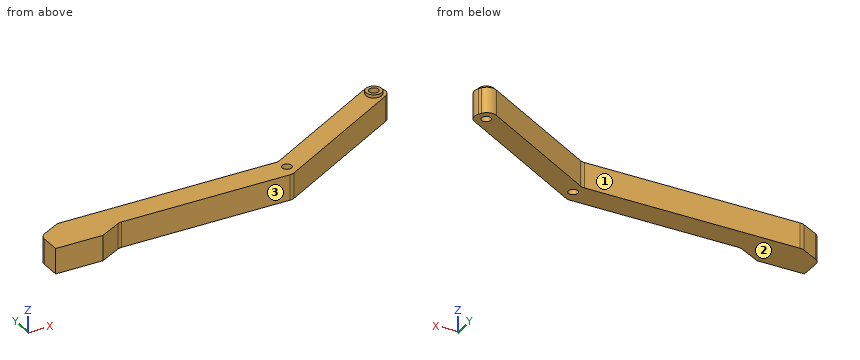
from build123d import *

# Parameters (mm, degrees)
SKETCH_1_R      = 1.5
EXTRUDE_1_DEPTH = 8
FILLET_1_R      = 3
SKETCH_2_R      = 2.5
SKETCH_2_R_2    = 1.5
EXTRUDE_2_DEPTH = 1


with BuildPart() as part:
    # 草图1 → 凸台-拉伸1 (new body)
    with BuildSketch(Plane.XY):
        Polygon((-7.5, 4), (-7.5, -4), (7.5, -4), (15, 0), (70, 0), (116.765371804, 27), (113.301270189, 33), (70, 8), (0, 8), align=None)
        with Locations((112.0368731, 28.27)):
            Circle(SKETCH_1_R, mode=Mode.SUBTRACT)
        with Locations((70.727461339, 4.42)):
            Circle(SKETCH_1_R, mode=Mode.SUBTRACT)
    extrude(amount=EXTRUDE_1_DEPTH)

    # 圆角1
    fillet_1_edges = [part.edges().sort_by_distance(p)[0] for p in [
        (-7.5, 4, 4),
        (0, 8, 4),
        (70, 8, 4),
        (113.301270189, 33, 4),
        (116.765371804, 27, 4),
        (70, 0, 4),
        (15, 0, 4),
    ]]
    fillet(fillet_1_edges, radius=FILLET_1_R)

    # 草图2 → 凸台-拉伸2 (add)
    with BuildSketch(Plane.XY.offset(8)):
        with Locations((112.0368731, 28.27)):
            Circle(SKETCH_2_R)
        with Locations((112.0368731, 28.27)):
            Circle(SKETCH_2_R_2, mode=Mode.SUBTRACT)
    extrude(amount=EXTRUDE_2_DEPTH)


solid = part.part
Check sheet for the modelled part. Datum: model origin and axes. Units: mm. Face numbers are marked on the shaded views. A direction names the side the tool comes from. Round coordinates to 2 decimals unless told otherwise and drop trailing zeros. Order: outer loops, then holes, each group sorted by start corner. A loop starts at its lowest first (then second) coordinate and runs counter-clockwise, first axis right, second up.
Q1. Scan lines: L1, parallel to Z at x = 38.5, y = 4; L2, parallel to Y at x = 1, z = 3.75; L3, parallel to X at y = 24, z = 5. Record each from-to range of solid material in increasing order.
Filled sheet:
L1: z = 0 to 8
L2: y = -4 to 8
L3: x = 97.71 to 111.57
Q2. Cross-section at A-A, the plane z = 5. Enter the section's corners in (x, y), plus the area to 3 significant figures.
Filled sheet:
outline: (-7.5, -4) - (7.5, -4) - (14.34, -0.35) arc R3 cw to (15.75, 0) - (69.2, 0) arc R3 ccw to (70.7, 0.4) - (114.17, 25.5) arc R3 ccw to (115.27, 29.6) - (114.8, 30.4) arc R3 ccw to (110.7, 31.5) - (70.7, 8.4) arc R3 cw to (69.2, 8) - (0.75, 8) arc R3 ccw to (-0.66, 7.65) - (-5.91, 4.85) arc R3 ccw to (-7.5, 2.2) - close; hole circle Ø3 at (70.73, 4.42); hole circle Ø3 at (112.04, 28.27)
area: 1,020 mm2
Q3. Cross-section at B-B, the plane y = 28.27. Enter the section's corners in (x, z), plus the area to 3 significant figures.
Filled sheet:
outline: (105.11, 0) - (110.54, 0) - (110.54, 9) - (109.54, 9) - (109.54, 8) - (105.11, 8) - close; (113.54, 0) - (115.66, 0) - (115.66, 8) - (114.54, 8) - (114.54, 9) - (113.54, 9) - close
area: 62.4 mm2
Q4. Set-up check for the marked faces 1, 2 and 3: record each of +Z, -Z, +X, -X, +Y, -Y from which the full face is reachable in a straight line by a thin tool's end or side.
Filled sheet:
face 1: +Z, -Z, -X, +Y
face 2: -Z, +X, -X, +Y, -Y
face 3: +Z, -Z, +X, -Y
Q5. Cross-section at D-D, the plane y = 21. Enter the section's corners in (x, z).
Filled sheet:
outline: (92.52, 0) - (106.37, 0) - (106.37, 8) - (92.52, 8) - close
Q6. Depth check by flat-ended pin: P1, Ø2, axis at x = 46.5, z = 7, coming from the -Y side; P2, Ø3, axis at y = 18, z = 7, coming from the +X side (3 decimals); P3, Ø3.5, axis at x = 70.73, y = 4.42, coming from the +Z side; P4, Ø8, axis at x = 91.5, y = 26, coming from the +Z side. Enter the tip coordinate at first touch or a pass-through.
Filled sheet:
P1: stops at y = 0
P2: stops at x = 103.775
P3: stops at z = 8
P4: passes through
Q7. Cross-section at C-C, the plane x = 89.5. Enter the section's corners in (y, z).
Filled sheet:
outline: (11.26, 0) - (19.26, 0) - (19.26, 8) - (11.26, 8) - close
